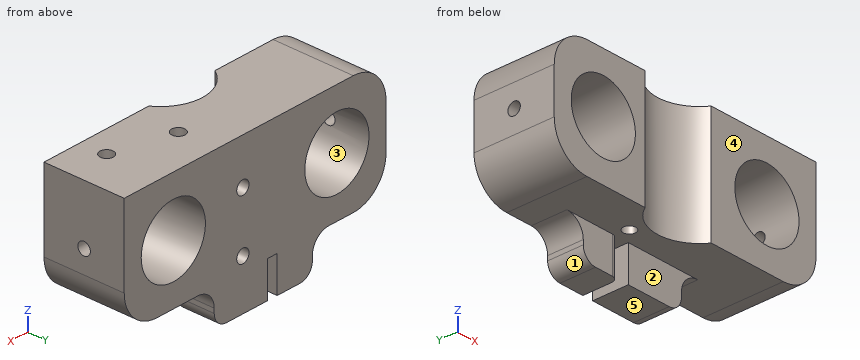
from build123d import *

# Parameters (mm, degrees)
BOX001_W        = 64
BOX001_H        = 18
BOX001_DEPTH    = 26
SKETCH010_R     = 7.85
POCKET001_DEPTH = 18.001
SKETCH011_W     = 24
SKETCH011_H     = 8
PAD001_DEPTH    = 8
SKETCH017_R     = 9.4
POCKET003_DEPTH = 34.001
SKETCH019_R     = 1.5
POCKET005_DEPTH = 5
SKETCH022_R     = 1.4
POCKET008_DEPTH = 5
SKETCH023_R     = 1.4
POCKET009_DEPTH = 5
SKETCH025_R     = 1.4
POCKET010_DEPTH = 8
SKETCH028_R     = 1.5
POCKET013_DEPTH = 7.8
SKETCH024_W     = 2.4
SKETCH024_H     = 8.929814
POCKET014_DEPTH = 8
FILLET_R        = 4
FILLET001_R     = 3
FILLET002_R     = 1.5
FILLET003_R     = 8


with BuildPart() as part:
    # Box001 → Box001 (new body)
    with BuildSketch(Plane(origin=(0, 27, 0), x_dir=(1, 0, 0), z_dir=(0, 0, 1))):
        with Locations((32, 9)):
            Rectangle(BOX001_W, BOX001_H)
    extrude(amount=BOX001_DEPTH)

    # Sketch010 → Pocket001 (cut, through all)
    with BuildSketch(Plane.XZ.offset(-27)):
        with Locations((12, 13)):
            Circle(SKETCH010_R)
        with Locations((52, 13)):
            Circle(SKETCH010_R)
    extrude(amount=-POCKET001_DEPTH, mode=Mode.SUBTRACT)

    # Sketch011 → Pad001 (new body)
    with BuildSketch(Plane(origin=(0, 27, 0), x_dir=(1, 0, 0), z_dir=(0, 0, -1))):
        with Locations((30, -14)):
            Rectangle(SKETCH011_W, SKETCH011_H)
    extrude(amount=PAD001_DEPTH)

    # Sketch017 → Pocket003 (cut, through all)
    with BuildSketch(Plane(origin=(0, 27, 26), x_dir=(1, 0, 0), z_dir=(0, 0, 1))):
        with Locations((30.3, -4.8)):
            Circle(SKETCH017_R)
    extrude(amount=-POCKET003_DEPTH, mode=Mode.SUBTRACT)

    # Sketch019 → Pocket005 (cut)
    with BuildSketch(Plane(origin=(0, 27, 26), x_dir=(1, 0, 0), z_dir=(0, 0, 1))):
        with Locations((41.5, 9.5)):
            Circle(SKETCH019_R)
        with Locations((55, 5.8)):
            Circle(SKETCH019_R)
    extrude(amount=-POCKET005_DEPTH, mode=Mode.SUBTRACT)

    # Sketch022 → Pocket008 (cut)
    with BuildSketch(Plane(origin=(0, 27, 0), x_dir=(0, -1, 0), z_dir=(-1, 0, 0))):
        with Locations((-9, 13)):
            Circle(SKETCH022_R)
    extrude(amount=-POCKET008_DEPTH, mode=Mode.SUBTRACT)

    # Sketch023 → Pocket009 (cut)
    with BuildSketch(Plane(origin=(64, 27, 0), x_dir=(0, 1, 0), z_dir=(1, 0, 0))):
        with Locations((9, 13)):
            Circle(SKETCH023_R)
    extrude(amount=-POCKET009_DEPTH, mode=Mode.SUBTRACT)

    # Sketch025 → Pocket010 (cut)
    with BuildSketch(Plane(origin=(0, 27, 0), x_dir=(1, 0, 0), z_dir=(0, 0, -1))):
        with Locations((26, -7)):
            Circle(SKETCH025_R)
    extrude(amount=-POCKET010_DEPTH, mode=Mode.SUBTRACT)

    # Sketch028 → Pocket013 (cut)
    with BuildSketch(Plane(origin=(0, 45, 0), x_dir=(-1, 0, 0), z_dir=(0, 1, 0))):
        with Locations((-35, 3)):
            Circle(SKETCH028_R)
        with Locations((-35, 16)):
            Circle(SKETCH028_R)
    extrude(amount=-POCKET013_DEPTH, mode=Mode.SUBTRACT)

    # Sketch024 → Pocket014 (cut)
    with BuildSketch(Plane(origin=(0, 45, 0), x_dir=(-1, 0, 0), z_dir=(0, 1, 0))):
        with Locations((-27.8, -4.464907)):
            Rectangle(SKETCH024_W, SKETCH024_H)
    extrude(amount=-POCKET014_DEPTH, mode=Mode.SUBTRACT)

    # Fillet
    fillet_edges = [part.edges().sort_by_distance(p)[0] for p in [
        (18, 41, 0),
        (42, 41, 0),
    ]]
    fillet(fillet_edges, radius=FILLET_R)

    # Fillet001
    fillet001_edges = [part.edges().sort_by_distance(p)[0] for p in [
        (42, 41, -8),
        (18, 41, -8),
    ]]
    fillet(fillet001_edges, radius=FILLET001_R)

    # Fillet002
    fillet002_edges = [part.edges().sort_by_distance(p)[0] for p in [
        (26.6, 37, -4),
    ]]
    fillet(fillet002_edges, radius=FILLET002_R)

    # Fillet003
    fillet003_edges = [part.edges().sort_by_distance(p)[0] for p in [
        (64, 36, 0),
        (0, 36, 26),
        (0, 36, 0),
    ]]
    fillet(fillet003_edges, radius=FILLET003_R)


solid = part.part
Work out the finished part from the listing and answer in its coordinate system (mm). Face numbers are marked on the shaded views. A direction names the side the tool comes from. Give positions to 0.01 mm unless a question says otherwise; leave off trailing zeros. Write each loop counter-clockwise with the first axis right and the second up, starting at its lowest first coordinate (ties: lowest second). Pieces come first, ordered by that corner, then holes. Notation, with made-up numbers: (7, 36.5) - (49, 36.5) arc R27 ccw to (49, 65.5) - close; hole circle Ø1 at (-2, 88.5). An arc over 180 degrees is marked (long way). One line per item, written item: value. Start each with the question number.
1. Find section C-C (y = 30.5). Write down the section's boundary in (x, z), then the cut area to 3 significant figures.
2. For the marked faces 1 and 2, determine the directions among +Z, -Z, +X, -X, +Y, -Y from which every point of the face is accessible in a straight line to the end or side of a thin tool.
3. For a pull along Z with two mould halves and no side action, classify the marked faces 3, 4 and 5 as +Z half, -Z half, draft (parallel to the pull), parting line (faces both ways), or undercut.
4. Find section A-A (z = 13). Write down the section's boundary in (x, y), then the cut area to 3 significant figures.
5. Find section D-D (x = 52). Write down the section's boundary in (y, z), then the cut area to 3 significant figures.
6. Consider probe 1 along Z at (x, y) = (35, 42.25); probe 2 along Z at (x, y) = (12, 31); probe 3 along X at (y, z) = (36, 17). Determine where each line is inside the solid, lowest interval first.
7. Find section B-B (z = 7). Write down the section's boundary in (x, y).
8. Given pin 1 (9 mm diameter, centred on x = 21.5, y = 31.5, fed in from -Z); pin 2 (0.9 mm diameter, centred on x = 34.5, z = 2.5, fed in from +Y); pin 3 (5 mm diameter, centred on x = 37, z = 4, fed in from -Y); pin 4 (2 mm diameter, centred on y = 36, z = 13, fed in from +X), each flat-ended and moving along its own axis, determine where each tip first touches the part or whether it passes through.
Geometry results:
1. outline: (0, 8) arc R8 ccw to (8, 0) - (25.89, 0) - (25.89, 26) - (8, 26) arc R8 ccw to (0, 18) - close; (34.71, 0) - (56, 0) arc R8 ccw to (64, 8) - (64, 26) - (34.71, 26) - close; hole circle Ø15.7 at (12, 13); hole circle Ø15.7 at (52, 13)
1. area: 1,010 mm2
2. face 1: -Z, -X, +Y, -Y
2. face 2: -Z, +X, -X, -Y
3. face 3: undercut
3. face 4: draft
3. face 5: -Z half
4. outline: (0, 27) - (4.15, 27) - (4.15, 34.6) - (0, 34.6) - close; (0, 37.4) - (4.15, 37.4) - (4.15, 45) - (0, 45) - close; (19.85, 27) - (22.22, 27) arc R9.4 cw to (38.38, 27) - (44.15, 27) - (44.15, 45) - (19.85, 45) - close; (59.85, 27) - (64, 27) - (64, 34.6) - (59.85, 34.6) - close; (59.85, 37.4) - (64, 37.4) - (64, 45) - (59.85, 45) - close
4. area: 511 mm2
5. outline: (27, 0) - (45, 0) - (45, 5.15) - (27, 5.15) - close; (27, 20.85) - (45, 20.85) - (45, 26) - (27, 26) - close
5. area: 185 mm2
6. probe 1: -8 to 1.5, 4.5 to 14.5, 17.5 to 26
6. probe 2: 0 to 5.15, 20.85 to 26
6. probe 3: 0 to 5.25, 18.75 to 45.25, 58.75 to 64
7. outline: (0.06, 27) - (6.94, 27) - (6.94, 45) - (0.06, 45) - close; (17.06, 27) - (22.22, 27) arc R9.4 cw to (38.38, 27) - (46.94, 27) - (46.94, 45) - (17.06, 45) - close; (57.06, 27) - (63.94, 27) - (63.94, 45) - (57.06, 45) - close; hole circle Ø2.8 at (26, 34)
8. pin 1: z = 0
8. pin 2: y = 37.2
8. pin 3: y = 27
8. pin 4: x = 44.21
